Read the model definition and answer for the solid it produces. Units are mm, in the model's axes. A direction names the side the tool comes from. Give positions to 0.01 mm unless a question says otherwise; leave off trailing zeros. Loops run counter-clockwise (first coordinate to the right, second up) from the corner with the lowest first, then second, coordinate; pieces in that order, holes last.
(1) Straight lines are drawn through the part: probe 1 along Y at (x, z) = (0, 3.75); probe 2 along Z at (x, y) = (0.75, -0.5); probe 3 along X at (y, z) = (1.75, 2.5). For each, find the intervals that lie inside material, in ascending order.
(2) Each of these flat-tipped pins is pushed along its axis until it touches: P1, Ø2, axis at x = 1.5, z = 5.5, coming from the -Y side; P2, Ø3, axis at x = 1.5, z = 2, coming from the +Y side; P3, Ø2.5, axis at x = -0.5, y = 1, coming from the +Z side. Where does it stop, or does it pass through?
(3) Which of the six approach directions +Z, -Z, +X, -X, +Y, -Y give full straight-line access (tool end or side, diameter ignored) to faces 4 (the face through (0, 0, 0)), 5 (the face through (-2, 2, 8)), 6 (the face through (3.106, -2.218, 1.374))?
(4) Find section C-C, the plane x = 0. Write down the section's boundary in (y, z).
(5) Find section D-D, the plane x = 3.5. Write down the section's boundary in (y, z), then the cut area to 3 significant figures.
(6) Find section B-B, the plane z = 1.75. Write down the section's boundary in (x, y).
(7) Determine the mould class of faces 1 (the face through (-3, 0, 4)), 2 (the face through (0, 0, -0.5)), 3 (the face through (-0.54, -2.44, 4.06)) for opening direction Y: pulls with the +Y half, pulls with the -Y half, needs draft (parallel to the pull), parting line crosses it, or undercut.
```python
from build123d import *

# Parameters (mm, degrees)
SKETCH2_R                = 3
SKETCH2_R_2              = 2.5
BOSS_EXTRUDE1_DEPTH      = 8
BOSS_EXTRUDE6_REACH      = 11.394
BOSS_EXTRUDE6_END_RADIUS = 3
SKETCH7_R                = 2.5
SKETCH7_R_2              = 1.539100033
SKETCH8_R                = 3
BOSS_EXTRUDE7_DEPTH      = 0.5


with BuildPart() as part:
    # Sketch2 → Boss-Extrude1 (new body)
    with BuildSketch(Plane.XY.offset(8)):
        Circle(SKETCH2_R)
        Circle(SKETCH2_R_2, mode=Mode.SUBTRACT)
    extrude(amount=-BOSS_EXTRUDE1_DEPTH)

    # Boss-Extrude6: up to this cylinder (the profile starts outside it)
    boss_extrude6_end = Plane(origin=(0, 0, 4.957209), z_dir=(0, 0, 1)) * Cylinder(BOSS_EXTRUDE6_END_RADIUS, 29.788, mode=Mode.PRIVATE)
    # Sketch7 → Boss-Extrude6 (add, up to the surface)
    with BuildSketch(Plane(origin=(4, 0, 2.500950228), x_dir=(0, 0, -1), z_dir=(1, 0, 0)), mode=Mode.PRIVATE) as boss_extrude6_sk1:
        with Locations((-0.026969657, 0)):
            Circle(SKETCH7_R)
        with Locations((-0.026969657, 0)):
            Circle(SKETCH7_R_2, mode=Mode.SUBTRACT)
    boss_extrude6_tool1 = extrude(boss_extrude6_sk1.sketch, amount=-BOSS_EXTRUDE6_REACH, mode=Mode.PRIVATE) - boss_extrude6_end
    add(boss_extrude6_tool1.solids().sort_by_distance((4, 0, 4.957209))[0])

    # Sketch8 → Boss-Extrude7 (add)
    with BuildSketch(Plane(origin=(0, 0, 0), x_dir=(-1, 0, 0), z_dir=(0, 0, -1))):
        with Locations(Location((0, 0, 0), (0, 0, 180))):
            Circle(SKETCH8_R)
    extrude(amount=BOSS_EXTRUDE7_DEPTH)

    # Fillet2: read off the stored shape, not the designer's step
    # Fillet2 outline → Fillet2 (revolve, cut)
    with BuildSketch(Plane.XZ):
        with BuildLine():
            Line((3, -0.5), (3, 0))
            ThreePointArc((3, 0), (2.853553391, -0.353553391), (2.5, -0.5))
            Line((2.5, -0.5), (3, -0.5))
        make_face()
    revolve(axis=Axis((0, 0, 0), (0, 0, 1)), mode=Mode.SUBTRACT)


solid = part.part
```
Entries:
1. probe 1: y = -3 to -2.5, 2.5 to 3
1. probe 2: z = -0.5 to 0
1. probe 3: x = -2.44 to -1.79, 1.79 to 4
2. P1: stops at y = -2.96
2. P2: stops at y = 3
2. P3: stops at z = 0
3. face 4: +Z
3. face 5: +Z, +X, -X, +Y, -Y
3. face 6: +X
4. outline: (-3, 0) arc R0.5 ccw to (-2.5, -0.5) - (2.5, -0.5) arc R0.5 ccw to (3, 0) - (3, 8) - (2.5, 8) - (2.5, 0) - (-2.5, 0) - (-2.5, 8) - (-3, 8) - close
5. outline: circle Ø5 at (0, 2.53); hole circle Ø3.08 at (0, 2.53)
5. area: 12.2 mm2
6. outline: (1.83, -2.38) - (4, -2.38) - (4, -1.33) - (2.69, -1.33) arc R3 ccw to (2.69, 1.33) - (4, 1.33) - (4, 2.38) - (1.83, 2.38) arc R3 ccw (long way) to start; hole circle Ø5 at (0, 0)
7. face 1: parting line crosses it
7. face 2: needs draft
7. face 3: undercut
